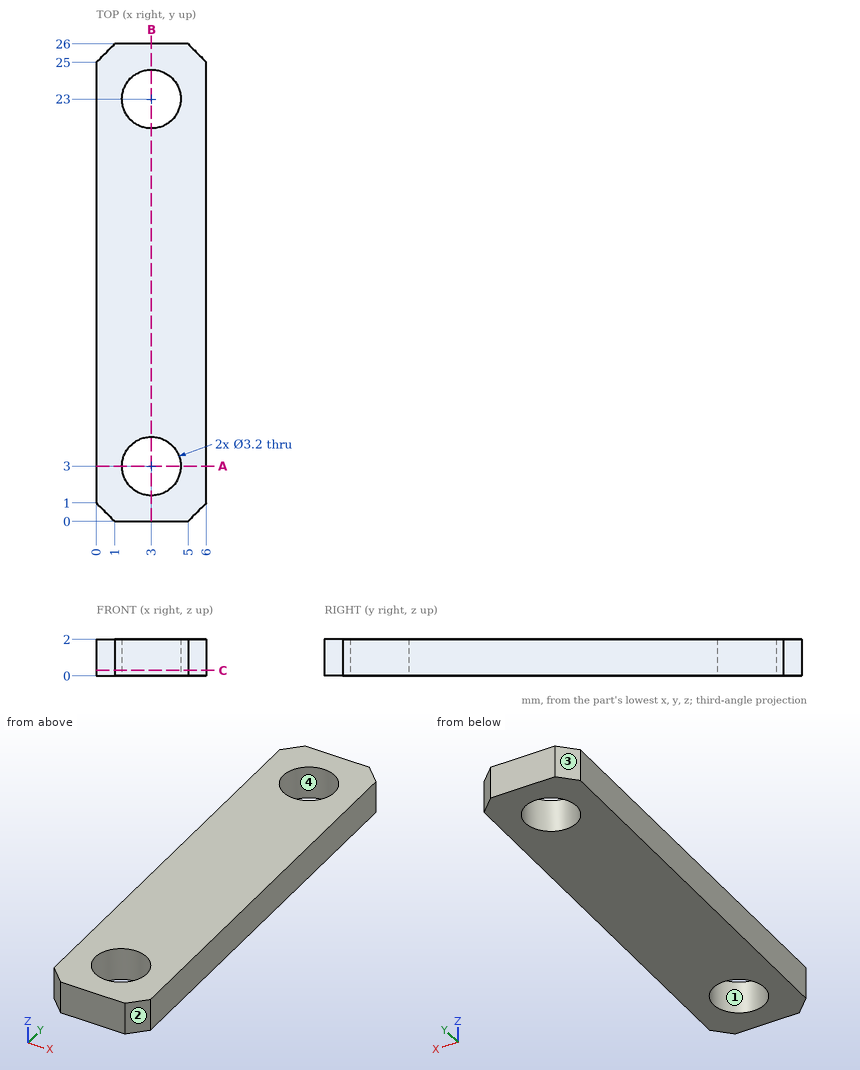
Study the drawing (mm; zero at the part's minimum x, y, z) and answer. Round coordinates to 2 decimals unless told otherwise and drop trailing zeros. Order: outer loops, then holes, each group sorted by start corner. A loop starts at its lowest first (then second) coordinate and runs counter-clockwise, first axis right, second up. Notation, with made-up numbers: M 60.25,71.25 L 113.25,71.25 A27 cw 113.25,108.25 Z; hole C 40.25,-4.75 d9. An arc over 180 degrees is marked long. One line per item, written item: value.
Q1. Find section B-B on x = 3. Write down the section's boundary in (y, z).
Derived:
outline: M 0,0 L 1.4,0 L 1.4,2 L 0,2 Z; M 4.6,0 L 21.4,0 L 21.4,2 L 4.6,2 Z; M 24.6,0 L 26,0 L 26,2 L 24.6,2 Z
Q2. Find section A-A on y = 3. Write down the section's boundary in (x, z), then the cut area to 3 significant figures.
Derived:
outline: M 0,0 L 1.4,0 L 1.4,2 L 0,2 Z; M 4.6,0 L 6,0 L 6,2 L 4.6,2 Z
area: 5.60 mm²
Q3. Determine the mould class of the marked faces 1, 2, 3 and 4 for opening direction X: released by +X, released by -X, zero draft, split by the parting line, or undercut.
Derived:
face 1: undercut
face 2: released by +X
face 3: released by -X
face 4: undercut
Q4. Find section C-C on z = 0.3. Write down the section's boundary in (x, y).
Derived:
outline: M 0,1 L 1,0 L 5,0 L 6,1 L 6,25 L 5,26 L 1,26 L 0,25 Z; hole C 3,3 d3.2; hole C 3,23 d3.2
Q5. Straight lines are drawn through the part: line 1 (Y direction, x = 3, z = 1.1); line 2 (X direction, y = 23, z = 1.3); line 3 (Y direction, x = 2.1, z = 1). For each, find the intervals that lie inside material, in ascending order.
Derived:
line 1: 0 to 1.4, 4.6 to 21.4, 24.6 to 26
line 2: 0 to 1.4, 4.6 to 6
line 3: 0 to 1.68, 4.32 to 21.68, 24.32 to 26
Q6. A flat-ended cylindrical pin translates along its axis: pin 1 (1.9 mm diameter, centred on x = 3, y = 3, fed in from -Z). Find the tip coordinate at first contact, or state that the pin passes through.
Derived:
pin 1: through
